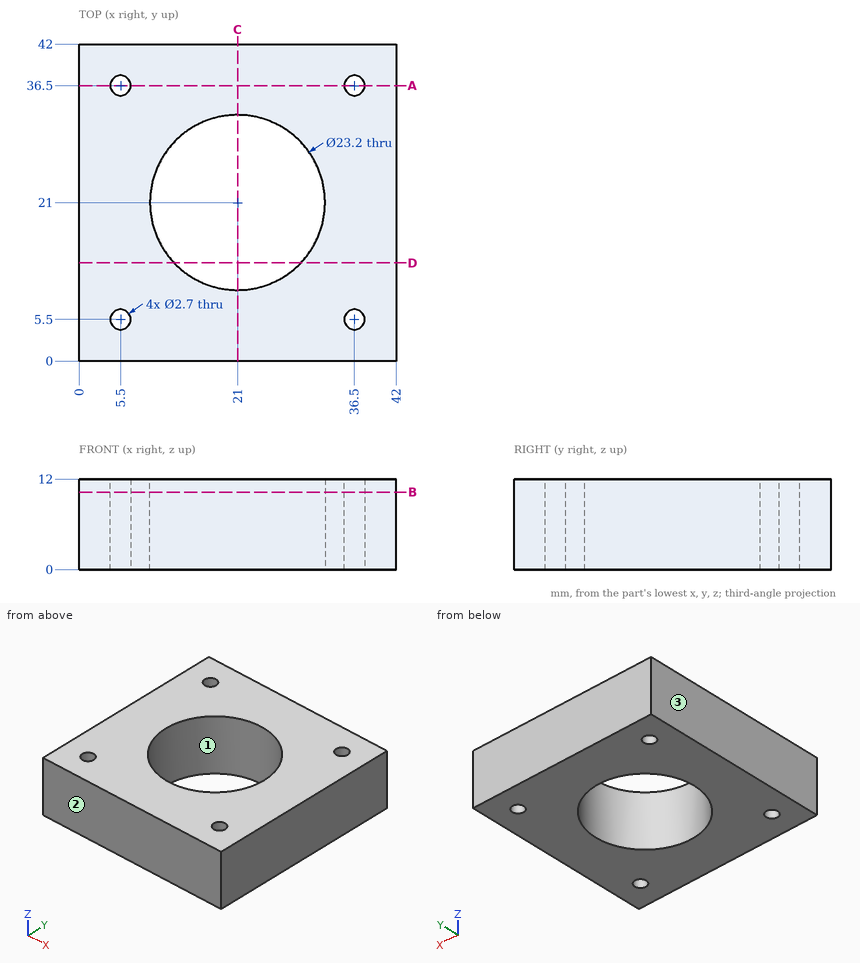
The drawing under review shows one solid part. Ordinate dimensions are in mm from its lowest x, y, z. Coordinates: 2 decimals unless noted, no trailing zeros. Order: outer loops, then holes, each group sorted by start corner. A loop starts at its lowest first (then second) coordinate and runs counter-clockwise, first axis right, second up. Notation, with made-up numbers: (55.25, 59) -> (111.25, 59) arc R21 cw to (111.25, 82) -> close; hole circle Ø7 at (38.25, 27). An arc over 180 degrees is marked (long way). Use CSV: the item, a comma, the result in double quotes. Start each with the question number.
Item 1: We need section D-D, the plane y = 13. Give the boundary of the cut face in (x, z), then the cut area to 3 significant figures.
Item 2: Draft analysis for pull direction Y (two halves, no side actions). For the marked faces 1, 2 and 3, state which applies: pulls with the +Y half, pulls with the -Y half, needs draft (parallel to the pull), parting line crosses it, or undercut.
Item 3: We need section A-A, the plane y = 36.5. Give the boundary of the cut face in (x, z), then the cut area to 3 significant figures.
Item 4: We need section B-B, the plane z = 10.25. Give the boundary of the cut face in (x, y).
Item 5: Wall thickness on probe 1 along Y at (x, z) = (5.5, 7); probe 2 along Y at (x, z) = (21, 6); probe 3 along X at (y, z) = (5, 7.75): over which ranges is each line inside the solid? List them lowest first.
Item 6: Insertion check: pin 1 (2.5 mm diameter, centred on x = 36.5, y = 5.5, fed in from +Z). The pin has a flat end and moves straight along its axis. Give the tip position at first contact, or say it passes through.
Item 7: We need section C-C, the plane x = 21. Give the boundary of the cut face in (y, z).
Derived:
1,outline,"(0, 0) -> (12.6, 0) -> (12.6, 12) -> (0, 12) -> close; (29.4, 0) -> (42, 0) -> (42, 12) -> (29.4, 12) -> close"
1,area,"302 mm^2"
2,face 1,"undercut"
2,face 2,"pulls with the -Y half"
2,face 3,"needs draft"
3,outline,"(0, 0) -> (4.15, 0) -> (4.15, 12) -> (0, 12) -> close; (6.85, 0) -> (35.15, 0) -> (35.15, 12) -> (6.85, 12) -> close; (37.85, 0) -> (42, 0) -> (42, 12) -> (37.85, 12) -> close"
3,area,"439 mm^2"
4,outline,"(0, 0) -> (42, 0) -> (42, 42) -> (0, 42) -> close; hole circle Ø2.7 at (5.5, 5.5); hole circle Ø2.7 at (5.5, 36.5); hole circle Ø23.2 at (21, 21); hole circle Ø2.7 at (36.5, 5.5); hole circle Ø2.7 at (36.5, 36.5)"
5,probe 1,"y = 0 to 4.15, 6.85 to 35.15, 37.85 to 42"
5,probe 2,"y = 0 to 9.4, 32.6 to 42"
5,probe 3,"x = 0 to 4.25, 6.75 to 35.25, 37.75 to 42"
6,pin 1,"passes through"
7,outline,"(0, 0) -> (9.4, 0) -> (9.4, 12) -> (0, 12) -> close; (32.6, 0) -> (42, 0) -> (42, 12) -> (32.6, 12) -> close"
